Part model, mm, in its own coordinate system. A direction names the side the tool comes from. Round coordinates to 2 decimals unless told otherwise and drop trailing zeros. Loops run counter-clockwise (first coordinate to the right, second up) from the corner with the lowest first, then second, coordinate; pieces in that order, holes last. Notation, with made-up numbers: M 23.25,23.25 L 47.25,23.25 A13 cw 47.25,45.25 Z; hole C -20.75,87.5 d1. An arc over 180 degrees is marked long. Put each result on its own line as item: value. Start each with the question number.
Autodesk Inventor part; units mm, degrees
ref_plane "YZ Plane" through (0, 0, 0) normal (1, 0, 0) x (0, 1, 0)
ref_plane "XZ Plane" through (0, 0, 0) normal (0, 1, 0) x (-1, 0, 0)
ref_plane "XY Plane" through (0, 0, 0) normal (0, 0, 1) x (1, 0, 0)
sketch "Sketch1" plane through (0, 0, 0) normal (0, 0, 1) x (1, 0, 0)
  line L0 (117.25, -7.54) -> (-117.25, -7.54)
  line L1 (-117.25, -7.54) -> (-117.25, 7.54)
  line L2 (-117.25, 7.54) -> (117.25, 7.54)
  line L3 (117.25, 7.54) -> (117.25, -7.54)
  line L4 (117.25, -7.54) -> (-117.25, 7.54) construction
  line L5 (-117.25, -7.54) -> (117.25, 7.54) construction
  point P0 (0, 0)
  dimension "d0" = 234.5
  dimension "d1" = 15.08
extrude "Extrusion1" add sketch "Sketch1" along normal blind 2.05
sketch "Sketch2" plane through (0, 0, 2.05) normal (0, 0, 1) x (1, 0, 0)
  line L0 (-117.25, -7.54) -> (117.25, -7.54)
  line L1 (117.25, -7.54) -> (117.25, 7.54)
  line L2 (-117.25, -7.54) -> (117.25, -7.54)
  line L3 (117.25, -7.54) -> (117.25, -5.49)
  line L4 (117.25, -5.49) -> (-117.25, -5.49)
  line L5 (-117.25, -5.49) -> (-117.25, -7.54)
  point P0 (0, 0)
  dimension "d4" = 2.05
extrude "Extrusion2" add sketch "Sketch2" along normal blind 13.03
sketch "Sketch3" plane through (-117.25, -5.49, 2.05) normal (0, 1, 0) x (1, 0, 0)
  circle A0 centre (23.75, -5.95) radius 1.6
  circle A1 centre (210.75, -5.95) radius 1.6
  line L0 (117.25, 2.05) -> (117.25, -13.2508)
  line L1 (0, 2.05) -> (234.5, 2.05)
  dimension "d7" = 93.5
  dimension "d8" = 93.5
  dimension "d9" = 8
  dimension "d10" = 8
  dimension "d13" = 3.2
  dimension "d14" = 3.2
extrude "Extrusion3" cut sketch "Sketch3" against normal blind 2.05
sketch "Sketch4" plane through (-117.25, -7.54, 0) normal (0, -1, 0) x (1, 0, 0)
  circle A0 centre (77.4621, 9.6496) radius 1.9
  point P0 (117.25, 0)
  dimension "d15" = 3.8
sketch "Sketch6" plane through (-117.25, -5.49, 2.05) normal (0, 1, 0) x (1, 0, 0)
  circle A0 centre (73.0521, -4.95) radius 1.75
  point P0 (117.25, 2.05)
extrude "Extrusion6" cut sketch "Sketch6" against normal blind 3
sketch "Sketch7" plane through (-117.25, -5.49, 2.05) normal (0, 1, 0) x (1, 0, 0)
  circle A0 centre (73.0521, -4.95) radius 1.75
  circle A1 centre (23.75, -5.95) radius 1.6
  circle A2 centre (210.75, -5.95) radius 1.6
  line L0 (0, 0) -> (234.5, 0)
  line L1 (0, 0) -> (0, -13.03)
  line L2 (234.5, -13.03) -> (0, -13.03)
  line L3 (234.5, 0) -> (234.5, -13.03)
  circle A3 centre (93.9521, -7.45) radius 1.6
  point P0 (117.25, 2.05)
extrude "Extrusion7" cut sketch "Sketch7" against normal blind 10 contours A3
sketch "Sketch8" plane through (0, 0, 2.05) normal (0, 0, 1) x (1, 0, 0)
  line L0 (-117.25, -5.49) -> (117.25, -5.49)
  line L1 (117.25, -5.49) -> (117.25, 7.54)
  line L2 (117.25, 7.54) -> (-117.25, 7.54)
  line L3 (-117.25, 7.54) -> (-117.25, -5.49)
  circle A0 centre (-93.2713, 0.46) radius 2.1
  circle A1 centre (93.7287, 0.46) radius 2.1
  point P0 (0, 0)
extrude "Extrusion8" cut sketch "Sketch8" against normal blind 10 contours A0 | A1
properties part number "L"
1. Cut at B-B, the plane z = 13. Give the cut face in (x, y), and give its area (3 significant figures).
2. Drop flat-ended pins along their axis: pin 1 (4 mm diameter, centred on x = 17, z = 10.5, fed in from +Y); pin 2 (3.5 mm diameter, centred on x = -93.27, y = 0.46, fed in from +Z). Give the stop position or say it passes through.
3. Wall check: L1, parallel to Z at x = -93.5, y = -6; L2, parallel to Z at x = -44, y = 3.75; L3, parallel to Y at x = -5, z = 13.25. Give the ranges that are in metal, low to high.
4. Cut at A-A, the plane x = 77. Give the cut face in (y, z), and give its area (3 significant figures).
5. Which spindle directions (+Z, -Z, +X, -X, +Y, -Y) get a long thin tool onto all of the face, cutting with end or side? Do faces 1 (the flat face through (-2, 0, 0)), 2 (the flat face through (-2, 1, 2.05)). Say none if no direction does.
6. Mould opens along X. For faces 3 (the flat face through (2, -5.49, 8)), 4 (the cylindrical face through (-91.33, -0.34, 1.04)), 5 (the cylindrical face through (95.67, -0.34, 1.04)), 6 (the flat face through (-117.25, -6, 4)) say: released by +X, released by -X, zero draft, split by the parting line, or undercut.
Results list:
1. outline: M -117.25,-7.54 L 117.25,-7.54 L 117.25,-5.49 L -117.25,-5.49 Z
1. area: 481 mm^2
2. pin 1: stops at y = -5.49
2. pin 2: passes through
3. L1: z = 0 to 6.4, 9.6 to 15.08
3. L2: z = 0 to 2.05
3. L3: y = -7.54 to -5.49
4. outline: M -7.54,0 L 7.54,0 L 7.54,2.05 L -5.49,2.05 L -5.49,15.08 L -7.54,15.08 Z
4. area: 57.6 mm^2
5. face 1: -Z, +X, -X, +Y, -Y
5. face 2: +Z, +X, -X, +Y
6. face 3: zero draft
6. face 4: undercut
6. face 5: undercut
6. face 6: released by -X
